Could you check a few things on this model? Use its own coordinates, in mm. A direction names the side the tool comes from. Give positions to 0.01 mm unless a question says otherwise; leave off trailing zeros. Order: outer loops, then holes, each group sorted by start corner. A loop starts at its lowest first (then second) coordinate and runs counter-clockwise, first axis right, second up. Notation, with made-up numbers: M 43,31.5 L 100,31.5 A20 ccw 100,60.5 Z; hole C 76.5,-29 d8. An arc over 180 degrees is marked long. Use a Markdown table: item, result. Add a question column.
```python
from build123d import *

# Parameters (mm, degrees)
F1_DEPTH      = 10
F1_DEPTH_BACK = 10
F2_DEPTH      = 2
F2_DEPTH_BACK = 2
F3_R          = 3


with BuildPart() as f1:
    # F0 (on Top) → F1 (new body, two sides)
    with BuildSketch(Plane.XY) as f1_sk:
        Polygon((-59.2774198156, 20), (-59.2774198156, 0), (59.2774198156, 0), (62.5326499412, 0), (62.5326499412, 14.9209070821), (60.5326499412, 14.9209070821), (59.2774198156, 5), align=None)
        with BuildLine():
            Line((-57.2774198156, 5.487030372), (-57.2774198156, 14.937681146))
            ThreePointArc((-57.2774198156, 14.937681146), (-56.0362820698, 16.769830707), (-53.888312773, 17.3022054044))
            Line((-53.888312773, 17.3022054044), (-53.8724083408, 17.3001931164))
            Line((-53.8724083408, 17.3001931164), (-23.888312773, 13.5064936359))
            ThreePointArc((-23.888312773, 13.5064936359), (-23.1661479004, 13.4609895281), (-22.4554066533, 13.3251970152))
            Line((-22.4554066533, 13.3251970152), (-5.8840475922, 11.2285269283))
            ThreePointArc((-5.8840475922, 11.2285269283), (-5.109007468, 11.1961309679), (-4.3503218976, 11.0344742393))
            Line((-4.3503218976, 11.0344742393), (42.1202175885, 5.1548484521))
            ThreePointArc((42.1202175885, 5.1548484521), (43.5106359985, 3.5774242261), (42.1202175885, 2))
            Line((42.1202175885, 2), (-5.4933972374, 2))
            ThreePointArc((-5.4933972374, 2), (-5.6887224148, 1.9958677209), (-5.8840475922, 2))
            Line((-5.8840475922, 2), (-23.888312773, 2))
            Line((-23.888312773, 2), (-53.1070120633, 2))
            ThreePointArc((-53.1070120633, 2), (-55.756346344, 3.0688282572), (-57.2774198156, 5.487030372))
        make_face(mode=Mode.SUBTRACT)
    extrude(amount=F1_DEPTH)
    extrude(f1_sk.sketch, amount=-F1_DEPTH_BACK)

    # F0 (on Top) → F2 (join, two sides)
    with BuildSketch(Plane.XY) as f2_sk:
        with BuildLine():
            ThreePointArc((-22.4554066533, 13.3251970152), (-18.1805700628, 7.0310819454), (-23.888312773, 2))
            Line((-23.888312773, 2), (-5.8840475922, 2))
            ThreePointArc((-5.8840475922, 2), (-10.3071181581, 6.6142634641), (-5.8840475922, 11.2285269283))
            Line((-5.8840475922, 11.2285269283), (-22.4554066533, 13.3251970152))
        make_face()
    extrude(amount=F2_DEPTH)
    extrude(f2_sk.sketch, amount=-F2_DEPTH_BACK)

    # F3
    f3_edges = [f1.edges().sort_by_distance(p)[0] for p in [
        (62.53265, 0, 0),
        (-59.27742, 0, 0),
        (-59.27742, 20, 0),
        (59.27742, 5, 0),
        (61.53265, 14.920907, -10),
        (61.53265, 14.920907, 10),
    ]]
    fillet(f3_edges, radius=F3_R)


solid = f1.part
```
1) We'd pull the mould along X, two halves only. Please class faces 4 (the face through (-59.277, 10, 0)), 5 (the face through (-14.286, 12.292, 6.056)), 6 (the face through (1, 11, 10)), 7 (the face through (-18.497, 9.761, 0.047)): pulls with the +X half, pulls with the -X half, needs draft (parallel to the pull), parting line crosses it, or undercut.
2) Suppose I cut it at B-B on x = 3.5. Please give me the cut outline in (y, z), and give its area (3 significant figures).
3) Suppose I cut it at C-C on z = -8. Please give me the cut outline in (x, y), and give its area (3 significant figures).
4) For pin 1 (3.5 mm diameter, centred on x = -15.5, y = 5.5, fed in from +Z); pin 2 (10.5 mm diameter, centred on x = -5.69, y = 6.61, fed in from +Z); pin 3 (5 mm diameter, centred on x = 19.5, z = 0, fed in from +Y); pin 4 (2 mm diameter, centred on x = -45, z = -1.5, fed in from +Y), each with a flat end and sliding along its axis, tell me the tip position at first contact or that it passes through.
5) For faces 1 (the face through (43.51, 3.61, 0.14)), 2 (the face through (-29, 2, 0)), 3 (the face through (62, 14.921, 0)), which set-ups out of +Z, -Z, +X, -X, +Y, -Y let a thin tool reach every point of the face, with its end or its side?
6) Suppose I cut it at A-A on z = -0.75. Please give me the cut outline in (x, y).
7) Please list where these lines run through material, in increasing order: line 1 (Y direction, x = 26, z = 5.25); line 2 (Y direction, x = -8.5, z = 6); line 3 (Z direction, x = -11, y = 11). Write a range as from..to.
Values found:
| question | item | result |
|---|---|---|
| 1 | face 4 | pulls with the -X half |
| 1 | face 5 | undercut |
| 1 | face 6 | needs draft |
| 1 | face 7 | undercut |
| 2 | outline | M 0,-10 L 2,-10 L 2,10 L 0,10 Z; M 10.04,-10 L 12.06,-10 L 12.06,10 L 10.04,10 Z |
| 2 | area | 80.3 mm^2 |
| 3 | outline | M -59.28,3 A3 ccw -56.28,0 L 59.53,0 A3 ccw 62.53,3 L 62.53,14.75 L 60.51,14.75 L 59.65,7.98 A3 cw 56.3,5.38 L -55.9,19.57 A3 ccw -59.28,16.6 Z; hole M -57.28,5.49 A4.64 ccw -53.11,2 L -5.88,2 A4.62 ccw -5.49,2 L 42.12,2 A1.59 ccw 42.12,5.15 L -4.35,11.03 A4.62 ccw -5.88,11.23 L -22.46,13.33 A5.75 ccw -23.89,13.51 L -53.89,17.3 A3.09 ccw -57.28,14.94 Z |
| 3 | area | 584 mm^2 |
| 4 | pin 1 | stops at z = 2 |
| 4 | pin 2 | stops at z = 10 |
| 4 | pin 3 | stops at y = 10.35 |
| 4 | pin 4 | stops at y = 18.32 |
| 5 | face 1 | +Z, -Z |
| 5 | face 2 | none |
| 5 | face 3 | +Z, -Z, +X, +Y |
| 6 | outline | M -59.28,3 A3 ccw -56.28,0 L 59.53,0 A3 ccw 62.53,3 L 62.53,14.92 L 60.53,14.92 L 59.65,7.98 A3 cw 56.3,5.38 L -55.9,19.57 A3 ccw -59.28,16.6 Z; hole M -57.28,5.49 A4.64 ccw -53.11,2 L -23.89,2 A5.75 ccw -23.89,13.51 L -53.89,17.3 A3.09 ccw -57.28,14.94 Z; hole M -5.49,2 L 42.12,2 A1.59 ccw 42.12,5.15 L -4.35,11.03 A4.62 ccw long Z |
| 7 | line 1 | y = 0..2, 7.19..9.21 |
| 7 | line 2 | y = 0..2, 11.56..13.58 |
| 7 | line 3 | z = -2..2 |
